```python
from build123d import *

# Parameters (mm, degrees)
BOSS_EXTRUDE1_DEPTH      = 40
CUT_EXTRUDE1_DEPTH       = 121
SKETCH3_R                = 11
SKETCH3_R_2              = 8.1
CUT_EXTRUDE3_DEPTH       = 1.75
SKETCH5_R                = 15
CUT_EXTRUDE4_DEPTH       = 41.144838819
CUT_EXTRUDE7_DEPTH       = 116.5
SKETCH11_W               = 3
SKETCH11_H               = 33
BOSS_EXTRUDE2_DEPTH      = 12
BOSS_EXTRUDE2_DEPTH_BACK = 1.75
CUT_EXTRUDE8_REACH       = 51.224
BOSS_EXTRUDE3_DEPTH      = 3


with BuildPart() as part:
    # Sketch1 → Boss-Extrude1 (new body)
    with BuildSketch(Plane(origin=(0, 0, 0), x_dir=(1, 0, 0), z_dir=(0, 1, 0))):
        with BuildLine():
            Line((0, 0), (120, 0))
            Line((120, 0), (120, -43))
            ThreePointArc((120, -43), (60, -53), (0, -43))
            Line((0, -43), (0, 0))
        make_face()
    extrude(amount=BOSS_EXTRUDE1_DEPTH)

    # Sketch2 → Cut-Extrude1 (cut, through all)
    with BuildSketch(Plane(origin=(120, 0, 0), x_dir=(0, 0, -1), z_dir=(1, 0, 0))):
        Polygon((-12.593217306, 40), (-53, 25.293133837), (-53, 40), align=None)
    extrude(amount=-CUT_EXTRUDE1_DEPTH, mode=Mode.SUBTRACT)

    # Sketch3 → Cut-Extrude3 (cut)
    with BuildSketch(Plane(origin=(0, 39.368270888, 14.328878778), x_dir=(1, 0, 0), z_dir=(0, 0.939692621, 0.342020143))):
        with Locations((92, -18.169172911)):
            Circle(SKETCH3_R)
        with Locations((12, -16.281893201)):
            Circle(SKETCH3_R_2)
        Polygon((69, -32.152947642), (72, -32.152947642), (72, -27.152947642), (69, -27.152947642), (69, -14.152947642), (72, -14.152947642), (72, -9.152947642), (69, -9.152947642), (69, -4.152947642), (66, -4.152947642), (66, -37.152947642), (69, -37.152947642), align=None)
        Polygon((26.75, -32.152947642), (26.75, -37.152947642), (29.75, -37.152947642), (29.75, -4.152947642), (26.75, -4.152947642), (26.75, -9.152947642), (23.75, -9.152947642), (23.75, -14.152947642), (26.75, -14.152947642), (26.75, -27.152947642), (23.75, -27.152947642), (23.75, -32.152947642), align=None)
    extrude(amount=-CUT_EXTRUDE3_DEPTH, mode=Mode.SUBTRACT)

    # Sketch5 → Cut-Extrude4 (cut, through all)
    with BuildSketch(Plane(origin=(0, 37.723808801, 13.730343527), x_dir=(1, 0, 0), z_dir=(0, 0.939692621, 0.342020143))):
        with Locations((92, -18.169172911)):
            Circle(SKETCH5_R)
    extrude(amount=-CUT_EXTRUDE4_DEPTH, mode=Mode.SUBTRACT)

    # Sketch9 → Cut-Extrude7 (cut)
    with BuildSketch(Plane(origin=(118.25, 0, 0), x_dir=(0, 0, -1), z_dir=(1, 0, 0))):
        Polygon((-1.75, 0), (-1.75, 38.25), (-12.28464509, 38.25), (-41.900468263, 27.470721902), (-41.900468263, 0), align=None)
    extrude(amount=-CUT_EXTRUDE7_DEPTH, mode=Mode.SUBTRACT)

    # Sketch11 → Boss-Extrude2 (add, two sides)
    with BuildSketch(Plane(origin=(0, 39.368270888, 14.328878778), x_dir=(1, 0, 0), z_dir=(0, 0.939692621, 0.342020143))) as boss_extrude2_sk:
        with Locations((28.25, -20.652947642)):
            Rectangle(SKETCH11_W, SKETCH11_H)
        with Locations((67.5, -20.652947642)):
            Rectangle(SKETCH11_W, SKETCH11_H)
    extrude(amount=BOSS_EXTRUDE2_DEPTH)
    extrude(boss_extrude2_sk.sketch, amount=-BOSS_EXTRUDE2_DEPTH_BACK)

    # Cut-Extrude8: up to this face of the body (flat: up to its plane)
    cut_extrude8_end = Plane(part.part.faces().sort_by_distance((59.86605923, 33.016543965, 26.663447373))[0])
    # Sketch13 → Cut-Extrude8 (cut, up to the picked face)
    with BuildSketch(Plane.XZ, mode=Mode.PRIVATE) as cut_extrude8_sk1:
        with BuildLine():
            Line((1.75, 41.900468263), (118.25, 41.900468263))
            ThreePointArc((118.25, 41.900468263), (60, 51.396933895), (1.75, 41.900468263))
        make_face()
    cut_extrude8_tool1 = split(extrude(cut_extrude8_sk1.sketch, amount=-CUT_EXTRUDE8_REACH, mode=Mode.PRIVATE), bisect_by=cut_extrude8_end, keep=Keep.BOTH, mode=Mode.PRIVATE)
    add(cut_extrude8_tool1.solids().sort_by_distance((60, 0, 45.707612))[0], mode=Mode.SUBTRACT)

    # Sketch14 → Boss-Extrude3 (add)
    with BuildSketch(Plane.XZ):
        with BuildLine():
            Line((1.75, 1.75), (21.75, 1.75))
            Line((21.75, 1.75), (21.75, 47.363800311))
            ThreePointArc((21.75, 47.363800311), (11.672735446, 44.914982019), (1.75, 41.900468263))
            Line((1.75, 41.900468263), (1.75, 1.75))
        make_face()
        with BuildLine():
            Line((118.25, 1.75), (118.25, 41.900468263))
            ThreePointArc((118.25, 41.900468263), (108.327264554, 44.914982019), (98.25, 47.363800311))
            Line((98.25, 47.363800311), (98.25, 1.75))
            Line((98.25, 1.75), (118.25, 1.75))
        make_face()
    extrude(amount=-BOSS_EXTRUDE3_DEPTH)


solid = part.part
```
Can you work these out from the model? Positions are in its coordinate system, mm. A direction names the side the tool comes from. Coordinates: 2 decimals unless noted, no trailing zeros. Loops run counter-clockwise (first coordinate to the right, second up) from the corner with the lowest first, then second, coordinate; pieces in that order, holes last. Notation, with made-up numbers: (23.25, 79) - (55.25, 79) arc R15 ccw to (55.25, 89) - close; hole circle Ø7 at (27, 50.5). An arc over 180 degrees is marked (long way). Use a Markdown table: item, result.
Item 1: Will these pins go through, and if not, where does the flat tip stop? pin 1 (10 mm diameter, centred on x = 111.5, z = 15.5, fed in from +Y); pin 2 (5 mm diameter, centred on x = 78, z = 43, fed in from -Y); pin 3 (3 mm diameter, centred on x = 87.5, y = 6, fed in from +Z).
Numbers:
| item | result |
|---|---|
| pin 1 | stops at y = 40 |
| pin 2 | stops at y = 26.16 |
| pin 3 | stops at z = 51.16 |
Item 2: I want a section at B-B on z = 10. Please give me the cut outline in (x, y).
Numbers:
| item | result |
|---|---|
| outline | (0, 0) - (21.75, 0) - (21.75, 3) - (1.75, 3) - (1.75, 38.25) - (118.25, 38.25) - (118.25, 3) - (98.25, 3) - (98.25, 0) - (120, 0) - (120, 40) - (0, 40) - close |
Item 3: I want a section at A-A on y = 10.5. Please give me the cut outline in (x, z).
Numbers:
| item | result |
|---|---|
| outline | (0, 0) - (120, 0) - (120, 43) arc R185 ccw to (0, 43) - close; hole (1.75, 1.75) - (118.25, 1.75) - (118.25, 41.9) arc R183.4 ccw to (1.75, 41.9) - close |
Item 4: I want a section at C-C on x = 111. Please give me the cut outline in (y, z), and give its area (3 significant figures).
Numbers:
| item | result |
|---|---|
| outline | (0, 0) - (40, 0) - (40, 12.59) - (27.9, 45.83) - (0, 45.83) - close; hole (3, 1.75) - (38.25, 1.75) - (38.25, 12.28) - (26.65, 44.16) - (3, 44.16) - close |
| area | 322 mm2 |
Item 5: I want a section at D-D on x = 50. Please give me the cut outline in (y, z), and give its area (3 significant figures).
Numbers:
| item | result |
|---|---|
| outline | (0, 0) - (40, 0) - (40, 12.59) - (25.39, 52.73) - (0, 52.73) - (0, 51.12) - (24.11, 51.12) - (38.25, 12.28) - (38.25, 1.75) - (0, 1.75) - close |
| area | 202 mm2 |
Item 6: For faces 1 (the face through (67.479, 43.507, 20.255)), 2 (the face through (98.25, 1, 25)), 3 (the face through (60.83, 13.543, 51.395)), which set-ups out of +Z, -Z, +X, -X, +Y, -Y let a thin tool reach every point of the face, with its end or its side?
Numbers:
| item | result |
|---|---|
| face 1 | +X, -X, +Y |
| face 2 | -Y |
| face 3 | none |
Item 7: If I drill on probe 1 along X at (y, z) = (27.5, 31); probe 2 along Y at (x, z) = (111.5, 4); probe 3 along X at (y, z) = (40, 37.5), over which ranges is the centre line in solid material (lowest first)? Write a range as from..to.
Numbers:
| item | result |
|---|---|
| probe 1 | x = 0..1.75, 118.25..120 |
| probe 2 | y = 0..3, 38.25..40 |
| probe 3 | x = 26.75..29.75, 66..69 |
Item 8: We'd pull the mould along Y, two halves only. Please class faces 4 (the face through (12, 3, 25)), 5 (the face through (61, 40, 6)), 6 (the face through (23.75, 28, 42)): released by +Y, released by -Y, zero draft, split by the parting line, or undercut.
Numbers:
| item | result |
|---|---|
| face 4 | undercut |
| face 5 | released by +Y |
| face 6 | zero draft |
